from build123d import *

# Parameters (mm, degrees)
F0_W     = 68.77514
F0_H     = 61.611074
F1_DEPTH = 25.4
F2_R     = 21.354475
F3_DEPTH = 13.462
F4_R     = 18.12526
F5_DEPTH = 60.452


with BuildPart() as f1:
    # F0 (on Front) → F1 (new body)
    with BuildSketch(Plane.XZ):
        Rectangle(F0_W, F0_H)
    extrude(amount=F1_DEPTH)

    # F2 (on face) → F3 (join)
    with BuildSketch(Plane.XZ):
        Circle(F2_R)
    extrude(amount=-F3_DEPTH)

    # F4 (on face) → F5 (cut)
    with BuildSketch(Plane(origin=(0, 13.462, 0), x_dir=(-1, 0, 0), z_dir=(0, 1, 0))):
        Circle(F4_R)
    extrude(amount=-F5_DEPTH, mode=Mode.SUBTRACT)


solid = f1.part
For this review, take the finished solid that the model builds, in its own axes (mm). A direction names the side the tool comes from. Coordinates: 2 decimals unless noted, no trailing zeros. Loops run counter-clockwise (first coordinate to the right, second up) from the corner with the lowest first, then second, coordinate; pieces in that order, holes last. Notation, with made-up numbers: (-11.75, 24) - (35.25, 24) arc R24 ccw to (35.25, 54) - close; hole circle Ø2 at (-37, -0.5). An arc over 180 degrees is marked (long way). Return JSON: item names as keys, results as strings.
Item 1: For line 1 (Z direction, x = 0, y = 3); line 2 (Z direction, x = 0, y = -11); line 3 (Y direction, x = 31, z = -10), list the stretches that pass through material, from the lowest coordinate up.
Determined:
{"line 1": "z = -21.35 to -18.13, 18.13 to 21.35", "line 2": "z = -30.81 to -18.13, 18.13 to 30.81", "line 3": "y = -25.4 to 0"}
Item 2: Take a section at D-D (x = 24.5). Give the boundary of the cut face in (y, z), then the cut area to 3 significant figures.
Determined:
{"outline": "(-25.4, -30.81) - (0, -30.81) - (0, 30.81) - (-25.4, 30.81) - close", "area": "1,560 mm2"}
Item 3: Take a section at A-A (x = 0). Give the boundary of the cut face in (y, z), then the cut area to 3 significant figures.
Determined:
{"outline": "(-25.4, -30.81) - (0, -30.81) - (0, -21.35) - (13.46, -21.35) - (13.46, -18.13) - (-25.4, -18.13) - close; (-25.4, 18.13) - (13.46, 18.13) - (13.46, 21.35) - (0, 21.35) - (0, 30.81) - (-25.4, 30.81) - close", "area": "731 mm2"}
Item 4: Take a section at C-C (y = -18). Give the boundary of the cut face in (x, z).
Determined:
{"outline": "(-34.39, -30.81) - (34.39, -30.81) - (34.39, 30.81) - (-34.39, 30.81) - close; hole circle Ø36.25 at (0, 0)"}
Item 5: Mouldability with a two-part tool opening along X and no side actions: class faces 1 (the cylindrical face through (3.9, -5.7, -17.7)), 2 (the cylindrical face through (-16.95, 6.64, -12.99)), 3 (the flat face through (-10, 13.462, -16)) as pulls with the +X half, pulls with the -X half, needs draft (parallel to the pull), parting line crosses it, or undercut.
Determined:
{"face 1": "undercut", "face 2": "parting line crosses it", "face 3": "needs draft"}
Item 6: For faces 4 (the flat face through (15, -25.4, 14)), 5 (the flat face through (-8, 0, 21)), list the 3-axis set-ups (+Z, -Z, +X, -X, +Y, -Y) from which the entire face can be reached by the end or side of a thin tool; tool diameter is ignored.
Determined:
{"face 4": "+Z, -Z, +X, -X, -Y", "face 5": "+Y"}
Item 7: Take a section at B-B (z = 0). Give the boundary of the cut face in (x, y), then the cut area to 3 significant figures.
Determined:
{"outline": "(-34.39, -25.4) - (-18.13, -25.4) - (-18.13, 13.46) - (-21.35, 13.46) - (-21.35, 0) - (-34.39, 0) - close; (18.13, -25.4) - (34.39, -25.4) - (34.39, 0) - (21.35, 0) - (21.35, 13.46) - (18.13, 13.46) - close", "area": "913 mm2"}
